Can you work these out from the model? Positions are in its coordinate system, mm. Face numbers are marked on the shaded views. A direction names the side the tool comes from. Give positions to 0.01 mm unless a question says otherwise; leave off trailing zeros. Loops run counter-clockwise (first coordinate to the right, second up) from the corner with the lowest first, then second, coordinate; pieces in that order, holes last. Notation, with made-up numbers: (28, 49.5) -> (45, 49.5) arc R30 cw to (45, 87.5) -> close; hole circle Ø4 at (-7.5, 40.5). An arc over 180 degrees is marked (long way). One line per question, with ' | ' between items.
from build123d import *

# Parameters (mm, degrees)
SKETCH1_R           = 40
BOSS_EXTRUDE1_DEPTH = 30
CUT_EXTRUDE2_DEPTH  = 40
SKETCH4_R           = 1.5
CUT_EXTRUDE3_DEPTH  = 40


with BuildPart() as part:
    # Sketch1 → Boss-Extrude1 (new body)
    with BuildSketch(Plane(origin=(0, 0, 0), x_dir=(1, 0, 0), z_dir=(0, 1, 0))):
        with Locations(Location((0, 0, 0), (0, 0, 270))):
            Circle(SKETCH1_R)
    extrude(amount=BOSS_EXTRUDE1_DEPTH)

    # Sketch2 → Cut-Extrude2 (cut)
    with BuildSketch(Plane(origin=(0, 30, 0), x_dir=(1, 0, 0), z_dir=(0, 1, 0))):
        with BuildLine():
            Line((-2.524208574, 29.893617564), (-4.690828974, 17.378035664))
            ThreePointArc((-4.690828974, 17.378035664), (-11.0328045, 14.222419796), (-15.666106265, 8.864147702))
            Line((-15.666106265, 8.864147702), (-28.175793715, 10.301681829))
            ThreePointArc((-28.175793715, 10.301681829), (-18.209434961, 23.841486497), (-2.524208574, 29.893617564))
        make_face()
        with BuildLine():
            Line((1.090682544, 29.980166971), (3.589212362, 17.638524729))
            ThreePointArc((3.589212362, 17.638524729), (10.117000938, 14.887790031), (15.077948188, 9.831351812))
            Line((15.077948188, 9.831351812), (27.650496433, 11.638300864))
            ThreePointArc((27.650496433, 11.638300864), (17.04757623, 24.685626277), (1.090682544, 29.980166971))
        make_face()
        with BuildLine():
            Line((28.849872599, 8.227080347), (17.884361498, 2.037060092))
            ThreePointArc((17.884361498, 2.037060092), (17.285454944, -5.021259539), (14.009513435, -11.301926089))
            Line((14.009513435, -11.301926089), (19.613155176, -22.700752059))
            ThreePointArc((19.613155176, -22.700752059), (28.745416497, -8.584930424), (28.849872599, 8.227080347))
        make_face()
        with BuildLine():
            Line((16.739519293, -24.895551688), (7.463930911, -16.379552355))
            ThreePointArc((7.463930911, -16.379552355), (0.565997728, -17.991099093), (-6.419592719, -16.816326273))
            Line((-6.419592719, -16.816326273), (-15.528899908, -25.668137207))
            ThreePointArc((-15.528899908, -25.668137207), (0.718068186, -29.99140507), (16.739519293, -24.895551688))
        make_face()
        with BuildLine():
            Line((-18.50428072, -23.613377459), (-13.271398505, -12.160180168))
            ThreePointArc((-13.271398505, -12.160180168), (-16.935649111, -6.097851195), (-17.977039929, 0.908864886))
            Line((-17.977039929, 0.908864886), (-29.210543127, 6.836970837))
            ThreePointArc((-29.210543127, 6.836970837), (-28.301625952, -9.950777279), (-18.50428072, -23.613377459))
        make_face()
    extrude(amount=-CUT_EXTRUDE2_DEPTH, mode=Mode.SUBTRACT)

    # Sketch4 → Cut-Extrude3 (cut)
    with BuildSketch(Plane(origin=(0, 30, 0), x_dir=(1, 0, 0), z_dir=(0, 1, 0))):
        with Locations(Location((0, 0, 0), (0, 0, 270))):
            Circle(SKETCH4_R)
    extrude(amount=-CUT_EXTRUDE3_DEPTH, mode=Mode.SUBTRACT)


solid = part.part
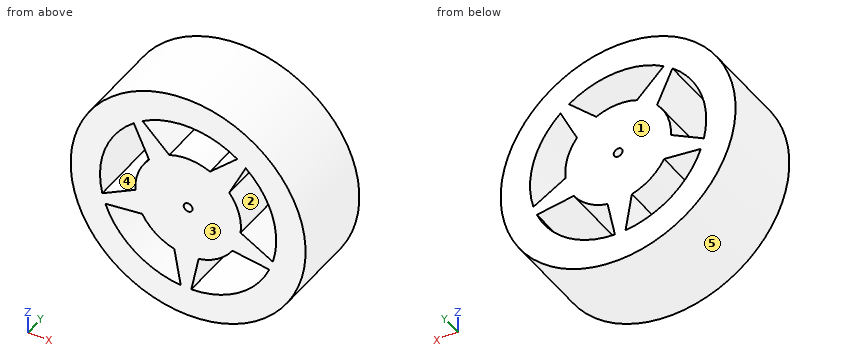
Q1. On a 3-axis mill with a long thin cutter (end or side, diameter ignored), from which of +Z, -Z, +X, -X, +Y, -Y can I reach the whole of each face in a straight line? I mean the marked faces 1 and 2. Say none if no direction works.
Entries:
face 1: +Z, -Z, +X, -X, +Y | face 2: +Y, -Y
Q2. If I drill on probe 1 along X at (y, z) = (17, 0); probe 2 along Z at (x, y) = (-6.5, 18.5); probe 3 along Z at (x, y) = (12, 22), over which ranges is the centre line in solid material (lowest first)? Write a range as from..to.
Entries:
probe 1: -40..-30, -18..-1.5, 1.5..18, 30..40 | probe 2: -39.47..-29.29, -16.79..16.89, 29.29..39.47 | probe 3: -38.16..-27.5, -13.42..20.54, 27.5..38.16
Q3. If we section it at C-C (y = 22.5): Write out the boundary of the cut face in (x, z).
Entries:
outline: circle Ø80 at (0, 0); hole (-29.21, -6.84) -> (-17.98, -0.91) arc R18 cw to (-13.27, 12.16) -> (-18.5, 23.61) arc R30 ccw to start; hole (-28.18, -10.3) arc R30 ccw to (-2.52, -29.89) -> (-4.69, -17.38) arc R18 cw to (-15.67, -8.86) -> close; hole (-15.53, 25.67) -> (-6.42, 16.82) arc R18 cw to (7.46, 16.38) -> (16.74, 24.9) arc R30 ccw to start; hole circle Ø3 at (0, 0); hole (1.09, -29.98) arc R30 ccw to (27.65, -11.64) -> (15.08, -9.83) arc R18 cw to (3.59, -17.64) -> close; hole (14.01, 11.3) arc R18 cw to (17.88, -2.04) -> (28.85, -8.23) arc R30 ccw to (19.61, 22.7) -> close
Q4. If we section it at A-A (x = 0): Write out the boundary of the cut face in (y, z), plus the area to 3 significant figures.
Entries:
outline: (0, -40) -> (30, -40) -> (30, -1.5) -> (0, -1.5) -> close; (0, 1.5) -> (30, 1.5) -> (30, 18) -> (0, 18) -> close; (0, 30) -> (30, 30) -> (30, 40) -> (0, 40) -> close | area: 1,950 mm²
Q5. If we section it at B-B (z = -21.5): Write out the boundary of the cut face in (x, y).
Entries:
outline: (-33.73, 0) -> (-20.92, 0) -> (-20.92, 30) -> (-33.73, 30) -> close; (-3.98, 0) -> (2.81, 0) -> (2.81, 30) -> (-3.98, 30) -> close; (20.92, 0) -> (33.73, 0) -> (33.73, 30) -> (20.92, 30) -> close
Q6. For pin 1 Ø6 at (y, z) = (16.5, 11) entering from -X; pin 2 Ø10 at (y, z) = (25.5, 11) entering from -X; pin 3 Ø6 at (x, y) = (-12, 19.5) entering from -Z, each with a flat end and sliding along its axis, tell me the tip position at first contact or that it passes through.
Entries:
pin 1: x = -39.19 | pin 2: x = -39.55 | pin 3: z = -38.97
Q7. If we mould it in two halves opening along Z, with no side actions, what happens to the marked faces 3, 4 and 5? For each: pulls with the +Z half, pulls with the -Z half, needs draft (parallel to the pull), parting line crosses it, or undercut.
Entries:
face 3: needs draft | face 4: undercut | face 5: parting line crosses it
Q8. If we section it at D-D (z = 21): Write out the boundary of the cut face in (x, y), plus the area to 3 significant figures.
Entries:
outline: (-34.04, 0) -> (-21.42, 0) -> (-21.42, 30) -> (-34.04, 30) -> close; (-17.31, 0) -> (-10.72, 0) -> (-10.72, 30) -> (-17.31, 30) -> close; (12.5, 0) -> (18.78, 0) -> (18.78, 30) -> (12.5, 30) -> close; (21.42, 0) -> (34.04, 0) -> (34.04, 30) -> (21.42, 30) -> close | area: 1,140 mm²
